from build123d import *

# Parameters (mm, degrees)
SKETCH1_R            = 6
BOSS_EXTRUDE4_DEPTH  = 5
BOSS_EXTRUDE5_DEPTH  = 30
BOSS_EXTRUDE6_DEPTH  = 30
SKETCH11_R           = 6
BOSS_EXTRUDE7_DEPTH  = 5
BOSS_EXTRUDE8_DEPTH  = 30
BOSS_EXTRUDE9_DEPTH  = 10
CUT_EXTRUDE2_REACH   = 126.008
SKETCH14_R           = 2.2
SKETCH16_W           = 25
SKETCH16_H           = 40
BOSS_EXTRUDE10_DEPTH = 52
CUT_EXTRUDE4_REACH   = 102.668
SKETCH18_R           = 19
SKETCH19_W           = 30
SKETCH19_H           = 5
BOSS_EXTRUDE11_DEPTH = 52
BOSS_EXTRUDE12_DEPTH = 50
BOSS_EXTRUDE14_REACH = 184.628
SKETCH22_W           = 10.000000149
SKETCH22_H           = 29.829068408
SKETCH26_R           = 2.15
SKETCH26_R_2         = 2.089802204
CUT_EXTRUDE6_DEPTH   = 33
CUT_EXTRUDE7_REACH   = 180.81
SKETCH27_R           = 3
SKETCH21_W           = 25
SKETCH21_H           = 10
SKETCH21_R           = 1.5
SKETCH21_W_2         = 50
BOSS_EXTRUDE15_DEPTH = 3
BOSS_EXTRUDE16_DEPTH = 5
BOSS_EXTRUDE17_START = -52
SKETCH30_R           = 30
SKETCH30_R_2         = 25
BOSS_EXTRUDE17_DEPTH = 52
SKETCH31_R           = 1.5
BOSS_EXTRUDE18_DEPTH = 3
CIRPATTERN1_COUNT    = 3
CIRPATTERN1_ANGLE    = 180


with BuildPart() as part:
    # Sketch1 → Boss-Extrude4 (new body)
    with BuildSketch(Plane(origin=(0, 0, 0), x_dir=(1, 0, 0), z_dir=(0, 1, 0))):
        with BuildLine():
            Line((0, 15), (60, 15))
            Line((60, 15), (60, -15))
            Line((60, -15), (0, -15))
            ThreePointArc((0, -15), (-15, 0), (0, 15))
        make_face()
        with Locations(Location((0, 0, 0), (0, 0, 270))):
            Circle(SKETCH1_R, mode=Mode.SUBTRACT)
    extrude(amount=BOSS_EXTRUDE4_DEPTH)

    # Sketch8 → Boss-Extrude5 (add)
    with BuildSketch(Plane.XY.offset(15)):
        Polygon((60, 0), (70, -10), (110, -10), (110, -5), (70, -5), (60, 5), align=None)
    extrude(amount=-BOSS_EXTRUDE5_DEPTH)

    # Sketch9 → Boss-Extrude6 (add)
    with BuildSketch(Plane.XY.offset(15)):
        Polygon((70, -10), (70, -21), (65, -21), (65, -5), align=None)
    boss_extrude6 = extrude(amount=-BOSS_EXTRUDE6_DEPTH)

    # Mirror3: Boss-Extrude6 across plane
    add(boss_extrude6.mirror(Plane(origin=(70, -21, -15), x_dir=(0, 0, 1), z_dir=(0, -1, 0))))



with BuildPart() as body_2:
    # Sketch11 → Boss-Extrude7 (new body)
    with BuildSketch(Plane(origin=(0, -42, 0), x_dir=(-1, 0, 0), z_dir=(0, -1, 0))):
        with BuildLine():
            Line((0, 15), (-60, 15))
            Line((-60, 15), (-60, -15))
            Line((-60, -15), (0, -15))
            ThreePointArc((0, -15), (15, 0), (0, 15))
        make_face()
        with Locations(Location((0, 0, 0), (0, 0, 270))):
            Circle(SKETCH11_R, mode=Mode.SUBTRACT)
    extrude(amount=BOSS_EXTRUDE7_DEPTH)


with BuildPart() as part_1:
    add(part.part)

    add(body_2.part)  # Boss-Extrude8 merges body 2
    # Sketch12 → Boss-Extrude8 (add)
    with BuildSketch(Plane(origin=(0, 0, -15), x_dir=(-1, 0, 0), z_dir=(0, 0, -1))):
        Polygon((-70, -32), (-65, -37), (-60, -42), (-60, -47), (-70, -37), (-110, -37), (-110, -32), align=None)
    extrude(amount=-BOSS_EXTRUDE8_DEPTH)

    # Sketch13 → Boss-Extrude9 (add)
    with BuildSketch(Plane(origin=(0, 0, -15), x_dir=(-1, 0, 0), z_dir=(0, 0, -1))):
        Polygon((-97, -10), (-97, -37), (-92, -37), (-92, -5), (-97, -5), align=None)
    extrude(amount=BOSS_EXTRUDE9_DEPTH)

    # Sketch14 → Cut-Extrude2 (cut, up to next)
    with BuildSketch(Plane(origin=(97, 0, 0), x_dir=(0, 0, -1), z_dir=(1, 0, 0)), mode=Mode.PRIVATE) as cut_extrude2_sk1:
        with Locations((19.3, -16.05)):
            Circle(SKETCH14_R)
    cut_extrude2_tool1 = extrude(cut_extrude2_sk1.sketch, amount=-CUT_EXTRUDE2_REACH, mode=Mode.PRIVATE) & part_1.part
    # Sketch14 → Cut-Extrude2 (cut, up to next)
    with BuildSketch(Plane(origin=(97, 0, 0), x_dir=(0, 0, -1), z_dir=(1, 0, 0)), mode=Mode.PRIVATE) as cut_extrude2_sk2:
        with Locations((19.3, -25.95)):
            Circle(SKETCH14_R)
    cut_extrude2_tool2 = extrude(cut_extrude2_sk2.sketch, amount=-CUT_EXTRUDE2_REACH, mode=Mode.PRIVATE) & part_1.part
    add(cut_extrude2_tool1.solids().sort_by_distance((97, -16.05, -19.3))[0], mode=Mode.SUBTRACT)
    add(cut_extrude2_tool2.solids().sort_by_distance((97, -25.95, -19.3))[0], mode=Mode.SUBTRACT)

    # Sketch16 → Boss-Extrude10 (add)
    with BuildSketch(Plane.XZ.offset(47)):
        with Locations((27.5, 35)):
            Rectangle(SKETCH16_W, SKETCH16_H)
    extrude(amount=-BOSS_EXTRUDE10_DEPTH)

    # Sketch18 → Cut-Extrude4 (cut, up to next)
    with BuildSketch(Plane(origin=(40, 0, 0), x_dir=(0, 0, -1), z_dir=(1, 0, 0)), mode=Mode.PRIVATE) as cut_extrude4_sk1:
        with Locations((-55, -21)):
            Circle(SKETCH18_R)
    cut_extrude4_tool1 = extrude(cut_extrude4_sk1.sketch, amount=-CUT_EXTRUDE4_REACH, mode=Mode.PRIVATE) & part_1.part
    add(cut_extrude4_tool1.solids().sort_by_distance((40, -21, 55))[0], mode=Mode.SUBTRACT)

    # Sketch19 → Boss-Extrude11 (add)
    with BuildSketch(Plane(origin=(110, 0, 0), x_dir=(0, 0, -1), z_dir=(1, 0, 0))):
        with Locations((0, -7.5)):
            Rectangle(SKETCH19_W, SKETCH19_H)
        with Locations((0, -34.5)):
            Rectangle(SKETCH19_W, SKETCH19_H)
    extrude(amount=BOSS_EXTRUDE11_DEPTH)

    # Sketch20 → Boss-Extrude12 (add)
    with BuildSketch(Plane(origin=(162, 0, 0), x_dir=(0, 0, -1), z_dir=(1, 0, 0))):
        with BuildLine():
            Line((-55, 5), (-55, -2))
            ThreePointArc((-55, -2), (-36, -21), (-55, -40))
            Line((-55, -40), (-55, -47))
            Line((-55, -47), (-30, -47))
            Line((-30, -47), (-15, -37))
            Line((-15, -37), (-15, -5))
            Line((-15, -5), (-30, 5))
            Line((-30, 5), (-55, 5))
        make_face()
    extrude(amount=-BOSS_EXTRUDE12_DEPTH)

    # Sketch22 → Boss-Extrude14 (add, up to next)
    with BuildSketch(Plane(origin=(0, 0, -15), x_dir=(-1, 0, 0), z_dir=(0, 0, -1)), mode=Mode.PRIVATE) as boss_extrude14_sk1:
        with Locations((-34.999999925, -27.085465796)):
            Rectangle(SKETCH22_W, SKETCH22_H)
    boss_extrude14_tool1 = extrude(boss_extrude14_sk1.sketch, amount=-BOSS_EXTRUDE14_REACH, mode=Mode.PRIVATE) - part_1.part
    add(boss_extrude14_tool1.solids().sort_by_distance((35, -27.085466, -15))[0])

    # Sketch26 → Cut-Extrude6 (cut)
    with BuildSketch(Plane(origin=(0, 5, 0), x_dir=(1, 0, 0), z_dir=(0, 1, 0))):
        with Locations(Location((34.000000507, -4.85, 0), (0, 0, 270))):
            Circle(SKETCH26_R)
        with Locations(Location((34.000000507, 4.85, 0), (0, 0, 270))):
            Circle(SKETCH26_R_2)
    extrude(amount=-CUT_EXTRUDE6_DEPTH, mode=Mode.SUBTRACT)

    # Sketch27 → Cut-Extrude7 (cut, up to next)
    with BuildSketch(Plane(origin=(0, 5, 0), x_dir=(1, 0, 0), z_dir=(0, 1, 0)), mode=Mode.PRIVATE) as cut_extrude7_sk1:
        with Locations(Location((34.000000507, 4.85, 0), (0, 0, 270))):
            Circle(SKETCH27_R)
    cut_extrude7_tool1 = extrude(cut_extrude7_sk1.sketch, amount=-CUT_EXTRUDE7_REACH, mode=Mode.PRIVATE) & part_1.part
    # Sketch27 → Cut-Extrude7 (cut, up to next)
    with BuildSketch(Plane(origin=(0, 5, 0), x_dir=(1, 0, 0), z_dir=(0, 1, 0)), mode=Mode.PRIVATE) as cut_extrude7_sk2:
        with Locations(Location((34.000000507, -4.85, 0), (0, 0, 270))):
            Circle(SKETCH27_R)
    cut_extrude7_tool2 = extrude(cut_extrude7_sk2.sketch, amount=-CUT_EXTRUDE7_REACH, mode=Mode.PRIVATE) & part_1.part
    add(cut_extrude7_tool1.solids().sort_by_distance((34.000001, 5, -4.85))[0], mode=Mode.SUBTRACT)
    add(cut_extrude7_tool2.solids().sort_by_distance((34.000001, 5, 4.85))[0], mode=Mode.SUBTRACT)

    # Sketch21 → Boss-Extrude15 (add)
    # profile 1 of 4: a face of its own
    with BuildSketch(Plane.XY.offset(55)):
        with Locations((27.5, 10)):
            Rectangle(SKETCH21_W, SKETCH21_H)
        with Locations((27.5, 10)):
            Circle(SKETCH21_R, mode=Mode.SUBTRACT)
    # profile 2 of 4: a face of its own
    with BuildSketch(Plane.XY.offset(55)):
        with Locations((27.5, -52)):
            Rectangle(SKETCH21_W, SKETCH21_H)
        with Locations((27.5, -52)):
            Circle(SKETCH21_R, mode=Mode.SUBTRACT)
    # profile 3 of 4: a face of its own
    with BuildSketch(Plane.XY.offset(55)):
        with Locations((137, 10)):
            Rectangle(SKETCH21_W_2, SKETCH21_H)
        with Locations((124.5, 10)):
            Circle(SKETCH21_R, mode=Mode.SUBTRACT)
        with Locations((149.5, 10)):
            Circle(SKETCH21_R, mode=Mode.SUBTRACT)
    # profile 4 of 4: a face of its own
    with BuildSketch(Plane.XY.offset(55)):
        with Locations((137, -52)):
            Rectangle(SKETCH21_W_2, SKETCH21_H)
        with Locations((124.5, -52)):
            Circle(SKETCH21_R, mode=Mode.SUBTRACT)
        with Locations((149.5, -52)):
            Circle(SKETCH21_R, mode=Mode.SUBTRACT)
    extrude(amount=-BOSS_EXTRUDE15_DEPTH)

    # Sketch28 → Boss-Extrude16 (add)
    with BuildSketch(Plane.XZ.offset(47)):
        with BuildLine():
            Line((0, 15), (0, 6))
            Line((0, 6), (-6, 6))
            Line((-6, 6), (-6, -6))
            Line((-6, -6), (0, -6))
            Line((0, -6), (0, -15))
            Line((0, -15), (-150, -15))
            Line((-150, -15), (-201.423008775, 46.28355545))
            ThreePointArc((-201.423008775, 46.28355545), (-178.836514307, 36.028181748), (-156.25001984, 46.28355545))
            Line((-156.25001984, 46.28355545), (-130, 15))
            Line((-130, 15), (0, 15))
        make_face()
    boss_extrude16 = extrude(amount=-BOSS_EXTRUDE16_DEPTH)

    # Mirror4: Boss-Extrude16 across plane
    add(boss_extrude16.mirror(Plane(origin=(0, -21, 0), x_dir=(0, 0, 1), z_dir=(0, -1, 0))))

    # Sketch30 → Boss-Extrude17 (add)
    with BuildSketch(Plane.XZ.offset(47).offset(BOSS_EXTRUDE17_START)):
        with Locations(Location((-178.836514307, 66.028181748, 0), (0, 0, 221.159253818))):
            Circle(SKETCH30_R)
        with Locations(Location((-178.836514307, 66.028181748, 0), (0, 0, 270))):
            Circle(SKETCH30_R_2, mode=Mode.SUBTRACT)
    extrude(amount=BOSS_EXTRUDE17_DEPTH)

    # Sketch31 → Boss-Extrude18 (add)
    with BuildSketch(Plane(origin=(0, 5, 0), x_dir=(1, 0, 0), z_dir=(0, 1, 0))):
        with BuildLine():
            Line((-160.566387425, -89.823190966), (-157.209024914, -92.955990517))
            ThreePointArc((-157.209024914, -92.955990517), (-149.591093676, -93.317472176), (-150.478249183, -85.742744428))
            Line((-150.478249183, -85.742744428), (-153.835611693, -82.609944877))
            ThreePointArc((-153.835611693, -82.609944877), (-156.902448834, -86.495149569), (-160.566387425, -89.823190966))
        make_face()
        with Locations(Location((-153.246771255, -89.906310873, 0), (0, 0, 270))):
            Circle(SKETCH31_R, mode=Mode.SUBTRACT)
    boss_extrude18 = extrude(amount=-BOSS_EXTRUDE18_DEPTH)

    # CirPattern1: Boss-Extrude18 ×3 about axis
    cirpattern1_axis = Axis((-178.836514307, 0, 66.028181748), (0, -1, 0))
    for i in range(1, CIRPATTERN1_COUNT):
        add(boss_extrude18.rotate(cirpattern1_axis, i * CIRPATTERN1_ANGLE / (CIRPATTERN1_COUNT - 1)))


solid = part_1.part
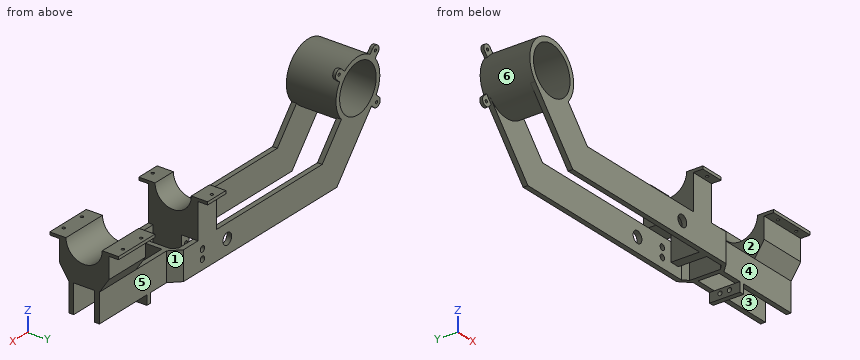
The listing builds one solid part. Answer for the finished solid, in the listing's coordinates (mm). Face numbers are marked on the shaded views. A direction names the side the tool comes from. Round coordinates to 2 decimals unless told otherwise and drop trailing zeros. Order: outer loops, then holes, each group sorted by start corner. A loop starts at its lowest first (then second) coordinate and runs counter-clockwise, first axis right, second up. Notation, with made-up numbers: M 85,-11.5 L 94,-11.5 A7 cw 94,-7.5 Z; hole C 42.25,30 d6. An arc over 180 degrees is marked long. Answer in a Markdown table with one row per item. Add a question column.
1) Which of the six approach directions +Z, -Z, +X, -X, +Y, -Y give full straight-line access (tool end or side, diameter ignored) to the marked faces 4, 5 and 6?
2) Consider line 1 along X through (y, z) = (-21.75, 4.85); line 2 along X through (y, z) = (-16, -14.5); line 3 along X through (y, z) = (-10, 20). Determine where each line is inside the solid, lowest interval first. Write a range as from..to.
3) Determine the mould class of the marked faces 1, 2 and 3 for opening direction X: pulls with the +X half, pulls with the -X half, needs draft (parallel to the pull), parting line crosses it, or undercut.
4) The part is cut by section B-B on z = 66. Determine the outline of the cut face in (x, y).
5) Flat-ended cylindrical pins translate along their axes: pin 1 Ø1 at (y, z) = (1.5, 50.5) entering from -X; pin 2 Ø24 at (y, z) = (-20, -4) entering from -X; pin 3 Ø8 at (x, y) = (114, -34.5) entering from +Z. Find the tip coordinate at first contact, or state that the pin passes through.
6) The part is cut by section A-A on x = -94. Determine the outline of the cut face in (y, z).
Findings below:
| question | item | result |
|---|---|---|
| 1 | face 4 | -Z, +X, -Y |
| 1 | face 5 | -Z, +X, +Y |
| 1 | face 6 | none |
| 2 | line 1 | x = 30..31.85, 36.15..40, 65..70 |
| 2 | line 2 | x = 30..40, 65..70 |
| 2 | line 3 | x = 15..40, 112..162 |
| 3 | face 1 | pulls with the +X half |
| 3 | face 2 | undercut |
| 3 | face 3 | needs draft |
| 4 | outline | M -208.84,-47 L -203.84,-47 L -203.84,5 L -208.84,5 Z; M -153.84,-47 L -148.84,-47 L -148.84,5 L -153.84,5 Z |
| 5 | pin 1 | stops at x = -204.8 |
| 5 | pin 2 | stops at x = 30 |
| 5 | pin 3 | stops at z = 47.6 |
| 6 | outline | M -47,-15 L -42,-15 L -42,15 L -47,15 Z; M 0,-15 L 5,-15 L 5,15 L 0,15 Z |
